```python
from build123d import *

# Parameters (mm, degrees)
BOSS_EXTRUDE1_DEPTH = 5.1
CHAMFER1_SIZE       = 2
FILLET1_R           = 1
SKETCH3_R           = 1
CUT_EXTRUDE1_DEPTH  = 5.1
SKETCH4_R           = 1
CUT_EXTRUDE2_DEPTH  = 5.1
SKETCH5_R           = 1.7
CUT_EXTRUDE3_DEPTH  = 1.4
SKETCH6_R           = 1.7
CUT_EXTRUDE4_DEPTH  = 1.4


with BuildPart() as part:
    # Sketch1 → Boss-Extrude1 (new body)
    with BuildSketch(Plane(origin=(0, 0, 0), x_dir=(1, 0, 0), z_dir=(0, 1, 0))):
        Polygon((0, 0), (0, 5.2), (-3, 5.2), (-3, -3), (5.2, -3), (5.2, 0), align=None)
    extrude(amount=BOSS_EXTRUDE1_DEPTH)

    # Chamfer1
    chamfer1_edges = [part.edges().sort_by_distance(p)[0] for p in [
        (-3, 2.55, 3),
    ]]
    chamfer(chamfer1_edges, length=CHAMFER1_SIZE)

    # Fillet1
    fillet1_edges = [part.edges().sort_by_distance(p)[0] for p in [
        (-1.5, 5.1, -5.2),
        (5.2, 5.1, 1.5),
        (5.2, 0, 1.5),
        (-1.5, 0, -5.2),
    ]]
    fillet(fillet1_edges, radius=FILLET1_R)

    # Sketch3 → Cut-Extrude1 (cut)
    with BuildSketch(Plane(origin=(0, 0, 0), x_dir=(0, 0, -1), z_dir=(1, 0, 0))):
        with Locations((2.5, 2.55)):
            Circle(SKETCH3_R)
    extrude(amount=-CUT_EXTRUDE1_DEPTH, mode=Mode.SUBTRACT)

    # Sketch4 → Cut-Extrude2 (cut)
    with BuildSketch(Plane(origin=(0, 0, 0), x_dir=(-1, 0, 0), z_dir=(0, 0, -1))):
        with Locations((-2.5, 2.55)):
            Circle(SKETCH4_R)
    extrude(amount=-CUT_EXTRUDE2_DEPTH, mode=Mode.SUBTRACT)

    # Sketch5 → Cut-Extrude3 (cut)
    with BuildSketch(Plane(origin=(0, 0, 0), x_dir=(-1, 0, 0), z_dir=(0, 0, -1))):
        with Locations((-2.5, 2.55)):
            Circle(SKETCH5_R)
    extrude(amount=-CUT_EXTRUDE3_DEPTH, mode=Mode.SUBTRACT)

    # Sketch6 → Cut-Extrude4 (cut)
    with BuildSketch(Plane.ZY.offset(3)):
        with Locations((-2.5, 2.55)):
            Circle(SKETCH6_R)
    extrude(amount=-CUT_EXTRUDE4_DEPTH, mode=Mode.SUBTRACT)


solid = part.part
```
CAD build for the part. Positions are in the model's coordinates, mm. A direction names the side the tool comes from. Round coordinates to 2 decimals unless told otherwise and drop trailing zeros. Write each loop counter-clockwise with the first axis right and the second up, starting at its lowest first coordinate (ties: lowest second). Pieces come first, ordered by that corner, then holes. Notation, with made-up numbers: M 39,43 L 56,43 A18 ccw 56,53 Z; hole C -27,-18.75 d3. An arc over 180 degrees is marked long. One line per question, with ' | ' between items.
1. Cut at A-A on x = 2.5. Write the cut outline in (y, z), and give its area (3 significant figures).
Working result:
outline: M 0,0 L 0.85,0 L 0.85,1.4 L 1.55,1.4 L 1.55,3 L 0,3 Z; M 3.55,1.4 L 4.25,1.4 L 4.25,0 L 5.1,0 L 5.1,3 L 3.55,3 Z | area: 7.34 mm2
2. Cut at D-D on z = -2.5. Write the cut outline in (x, y).
Working result:
outline: M -3,0 L 0,0 L 0,1.55 L -1.6,1.55 L -1.6,0.85 L -3,0.85 Z; M -3,4.25 L -1.6,4.25 L -1.6,3.55 L 0,3.55 L 0,5.1 L -3,5.1 Z
3. Pin check, flat tip, straight feed: pin 1 Ø1.7 at (y, z) = (2, -2.5) entering from -X. Stop position of the tip, or through.
Working result:
pin 1: x = -1.6
4. Probe L1, parallel to Y at x = 2.5, z = 1; L2, parallel to Y at x = -0.8, z = -2.5; L3, parallel to Z at x = 4.25, y = 3.5. List the from-to ranges inside material, lowest first. Write a range as from..to.
Working result:
L1: 0..0.85, 4.25..5.1 | L2: 0..1.55, 3.55..5.1 | L3: 0..3
5. Which spindle directions (+Z, -Z, +X, -X, +Y, -Y) get a long thin tool onto all of the face, cutting with end or side? Do faces 1 (the flat face through (2.1, 1.4, 1.4)), 2 (the flat face through (4, 1, 0)), 3 (the cylindrical face through (-2.31, 1.04, -1.72)). Say none if no direction does.
Working result:
face 1: -Z | face 2: -Z, +X, +Y, -Y | face 3: -X
6. Cut at B-B on z = 0.5. Write the cut outline in (x, y).
Working result:
outline: M -3,0 L 4.2,0 A1 ccw 5.2,1 L 5.2,4.1 A1 ccw 4.2,5.1 L -3,5.1 Z; hole C 2.5,2.55 d3.4
7. Cut at C-C on y = 1.75. Write the cut outline in (x, z), and give its area (3 significant figures).
Working result:
outline: M -3,-5.2 L 0,-5.2 L 0,-3.1 L -1.6,-3.1 L -1.6,-4 L -3,-4 Z; M -3,-1 L -1.6,-1 L -1.6,-1.9 L 0,-1.9 L 0,0 L 1,0 L 1,1.4 L 1.9,1.4 L 1.9,3 L -1,3 L -3,1 Z; M 3.1,1.4 L 4,1.4 L 4,0 L 5.2,0 L 5.2,3 L 3.1,3 Z | area: 26.0 mm2
8. Mould opens along Z. For faces 4 (the flat face through (-0.3, 5.1, 0.1)), 5 (the cylindrical face through (-0.79, 1.94, -1.71)), 6 (the flat face through (-1, 3, -5.2)) say: pulls with the +Z half, pulls with the -Z half, needs draft (parallel to the pull), parting line crosses it, or undercut.
Working result:
face 4: needs draft | face 5: undercut | face 6: pulls with the -Z half
